For this review, take the finished solid that the model builds, in its own axes (mm). A direction names the side the tool comes from. Coordinates: 2 decimals unless noted, no trailing zeros. Loops run counter-clockwise (first coordinate to the right, second up) from the corner with the lowest first, then second, coordinate; pieces in that order, holes last.
1. Machinability: for faces 1 (the face through (14, -1, 1)), 2 (the face through (19.6, 17.5, 2)), 3 (the face through (40, 87, 2)), which of the approach directions +Z, -Z, +X, -X, +Y, -Y give a long, thin tool a straight path to every point of the face, cutting with its end or side? Answer none if there is none.
2. Take a section at A-A, the plane y = 55.5. State the section outline as (x, z) points.
3. Take a section at D-D, the plane x = -5. State the section outline as (y, z) points.
4. Mouldability with a two-part tool opening along X and no side actions: class faces 4 (the face through (7, 29, 20)), 5 (the face through (-2, 66, 2)), 6 (the face through (-25.93, 28.6, 9.15)) as pulls with the +X half, pulls with the -X half, needs draft (parallel to the pull), parting line crosses it, or undercut.
5. Take a section at C-C, the plane y = 7. State the section outline as (x, z) points.
6. Clearance check with flat-ended pins moving along their axes: P1, Ø2, axis at x = 28, z = 11.5, coming from the +Y side; P2, Ø1.5, axis at x = -2.5, z = 6.5, coming from the -Y side; P3, Ø1.6, axis at y = -1, z = 1, coming from the -X side. State where each tip first meets the part, or that it passes through.
7. Take a section at B-B, the plane x = 13. State the section outline as (y, z) points.
8. To check wall thickness, follow probe 1 along X at (y, z) = (81.5, 0.5); probe 2 along Y at (x, z) = (39.3, 11); probe 3 along Z at (x, y) = (-25, 81). State the ranges of each line that lie inside material, in increasing order.
```python
from build123d import *

# Parameters (mm, degrees)
BOSS_EXTRUDE1_DEPTH      = 2
SKETCH2_W                = 22
SKETCH2_H                = 32
BOSS_EXTRUDE2_DEPTH      = 2
BOSS_EXTRUDE3_DEPTH      = 2
BOSS_EXTRUDE3_DEPTH_BACK = 2
SKETCH3_W                = 22
SKETCH3_H                = 60
BOSS_EXTRUDE4_DEPTH      = 18
BOSS_EXTRUDE4_DEPTH_BACK = 4
SKETCH4_W                = 21.5
SKETCH4_H                = 3
SKETCH4_W_2              = 18.5
SKETCH4_W_3              = 3
SKETCH4_H_2              = 59
BOSS_EXTRUDE5_DEPTH      = 22
FILLET1_R                = 10
CHAMFER1_SIZE            = 7
SKETCH6_R                = 1.5
CUT_EXTRUDE1_DEPTH       = 72
FILLET2_R                = 2
CHAMFER2_SIZE            = 10
CHAMFER3_SIZE            = 10
CHAMFER4_SIZE            = 5


with BuildPart() as part:
    # Sketch1 → Boss-Extrude1 (new body)
    with BuildSketch(Plane.XY):
        Polygon((-2, 30), (-2, -2), (4, -2), (4, 0), (0, 0), (0, 28), (18, 28), (18, 0), (14, 0), (14, -2), (20, -2), (20, 30), align=None)
    extrude(amount=BOSS_EXTRUDE1_DEPTH)

    # Sketch2 → Boss-Extrude2 (add)
    with BuildSketch(Plane(origin=(0, 0, 0), x_dir=(-1, 0, 0), z_dir=(0, 0, -1))):
        with Locations((-9, 14)):
            Rectangle(SKETCH2_W, SKETCH2_H)
    extrude(amount=BOSS_EXTRUDE2_DEPTH)

    # Sketch3 → Boss-Extrude3 (add, two sides: drawn at the far end of the back side and taken through both)
    with BuildSketch(Plane.XY.offset(-BOSS_EXTRUDE3_DEPTH_BACK)):
        with Locations((9, 60)):
            Rectangle(SKETCH3_W, SKETCH3_H)
    extrude(amount=BOSS_EXTRUDE3_DEPTH + BOSS_EXTRUDE3_DEPTH_BACK)

    # Sketch4 → Boss-Extrude4 (add, two sides: drawn at the far end of the back side and taken through both)
    with BuildSketch(Plane.XY.offset(2).offset(-BOSS_EXTRUDE4_DEPTH_BACK)):
        Polygon((-23.5, 28), (-23.5, 31), (-23.5, 90), (-26.5, 90), (-26.5, 28), align=None)
        with Locations((-12.75, 29.5)):
            Rectangle(SKETCH4_W, SKETCH4_H)
        with Locations((29.25, 29.5)):
            Rectangle(SKETCH4_W_2, SKETCH4_H)
        with Locations((40, 60.5)):
            Rectangle(SKETCH4_W_3, SKETCH4_H_2)
        Polygon((20, 31), (-2, 31), (-2, 28), (0, 28), (18, 28), (20, 28), align=None)
        with Locations((40, 29.5)):
            Rectangle(SKETCH4_W_3, SKETCH4_H)
    extrude(amount=BOSS_EXTRUDE4_DEPTH + BOSS_EXTRUDE4_DEPTH_BACK)

    # Sketch5 → Boss-Extrude5 (add)
    with BuildSketch(Plane(origin=(20, 0, 0), x_dir=(0, 0, -1), z_dir=(1, 0, 0))):
        with BuildLine():
            ThreePointArc((-2, 81), (-4.636038969, 74.636038969), (-11, 72))
            Line((-11, 72), (-2, 72))
            Line((-2, 72), (-2, 81))
        make_face()
        with BuildLine():
            Line((-2, 90), (-11, 90))
            ThreePointArc((-11, 90), (-4.636038969, 87.363961031), (-2, 81))
            Line((-2, 81), (-2, 90))
        make_face()
    extrude(amount=-BOSS_EXTRUDE5_DEPTH)

    # Fillet1
    # the kernel refuses this fillet: 10 mm, written as the material it adds along each edge
    with BuildSketch(Plane(origin=(20, 72, 2), x_dir=(0, 0, 1), z_dir=(-1, 0, 0))) as fillet1_piece_1_section:
        with BuildLine():
            CenterArc((10, -9.949874371), FILLET1_R, 95.739170477, 84.260829523)
            Line((0, -9.949874371), (-0.2, -9.949874371))
            Line((-0.2, -9.949874371), (-0.2, 0))
            Line((-0.2, 0), (0, 0.2))
            ThreePointArc((0, 0.2), (4.5, 0.2), (8.98, 0.198997487))
            Line((8.98, 0.198997487), (9, 0))
        make_face()
    fillet1_piece_1 = extrude(amount=22, mode=Mode.PRIVATE)
    fillet1_piece_1 = fillet1_piece_1 - Plane(origin=(9, 81, 11), x_dir=(0, 0, -1), z_dir=(1, 0, 0)) * Cylinder(9, 84, mode=Mode.PRIVATE)
    add(fillet1_piece_1)

    # Chamfer1
    chamfer1_edges = [part.edges().sort_by_distance(p)[0] for p in [
        (40, 90, -2),
        (-25, 90, -2),
        (-25, 90, 20),
        (40, 90, 20),
    ]]
    chamfer(chamfer1_edges, length=CHAMFER1_SIZE)

    # Sketch6 → Cut-Extrude1 (cut)
    with BuildSketch(Plane(origin=(41.5, 0, 0), x_dir=(0, 0, -1), z_dir=(1, 0, 0))):
        with Locations((-11, 81)):
            Circle(SKETCH6_R)
    extrude(amount=-CUT_EXTRUDE1_DEPTH, mode=Mode.SUBTRACT)

    # Fillet2
    fillet2_edges = [part.edges().sort_by_distance(p)[0] for p in [
        (38.5, 31, 9),
        (41.5, 28, 9),
        (-26.5, 28, 9),
        (-23.5, 31, 9),
    ]]
    fillet(fillet2_edges, radius=FILLET2_R)

    # Chamfer2
    chamfer2_edges = [part.edges().sort_by_distance(p)[0] for p in [
        (20, 28, 0),
        (-2, 28, 0),
    ]]
    chamfer(chamfer2_edges, length=CHAMFER2_SIZE)

    # Chamfer3
    chamfer3_edges = [part.edges().sort_by_distance(p)[0] for p in [
        (-2, 31, 0),
        (20, 31, 0),
    ]]
    chamfer(chamfer3_edges, length=CHAMFER3_SIZE)

    # Chamfer4
    chamfer4_edges = [part.edges().sort_by_distance(p)[0] for p in [
        (9, 31, 2),
    ]]
    chamfer(chamfer4_edges, length=CHAMFER4_SIZE)


solid = part.part
```
Results list:
1. face 1: +Z, -Y
1. face 2: +Z, +X, -X, -Y
1. face 3: -Z, +X, +Y
2. outline: (-26.5, -2) - (-23.5, -2) - (-23.5, 20) - (-26.5, 20) - close; (-2, -2) - (20, -2) - (20, 2) - (-2, 2) - close; (38.5, -2) - (41.5, -2) - (41.5, 20) - (38.5, 20) - close
3. outline: (21, -2) - (38, -2) - (38, 2) - (36, 2) - (31, 7) - (31, 20) - (28, 20) - (28, 2) - (21, 2) - close
4. face 4: needs draft
4. face 5: undercut
4. face 6: pulls with the -X half
5. outline: (-2, -2) - (20, -2) - (20, 2) - (18, 2) - (18, 0) - (0, 0) - (0, 2) - (-2, 2) - close
6. P1: stops at y = 31
6. P2: stops at y = 28
6. P3: stops at x = -2
7. outline: (-2, -2) - (90, -2) - (90, 11) arc R9 cw to (72, 11) arc R10 cw to (62.05, 2) - (36, 2) - (31, 7) - (31, 20) - (28, 20) - (28, 0) - (-2, 0) - close
8. probe 1: x = -26.5 to -23.5, -2 to 20, 38.5 to 41.5
8. probe 2: y = 28 to 79.5, 82.5 to 90
8. probe 3: z = -2 to 9.5, 12.5 to 20
